```python
from build123d import *

# Parameters (mm, degrees)
F0_R = 2.5
F2_R = 1.5
F5_R = 1.5
F8_R = 1


with BuildPart() as f3:
    # F0 (on Top) → F3 section 0
    with BuildSketch(Plane.XY):
        Circle(F0_R)
    # F2 (on offset) → F3 section 1
    with BuildSketch(Plane.XY.offset(8)):
        Circle(F2_R)
    loft()

    # F7: sweep along a path in F6
    with BuildLine(Plane.XZ) as f7_path:
        ThreePointArc((3.5, 10.7476860285), (1.5570925767, 9.9429074233), (0.7523139715, 8))
    # F5 (on offset) → F7 (sweep)
    with BuildSketch(Plane.YZ.offset(3.5)):
        with Locations((0, 11.5)):
            Circle(F5_R)
    sweep(path=f7_path.line)

    # F8
    f8_edges = [f3.edges().sort_by_distance(p)[0] for p in [
        (-1.06066, -1.06066, 8),
    ]]
    fillet(f8_edges, radius=F8_R)


solid = f3.part
```
Work out the finished part from the listing and answer in its coordinate system (mm). Give positions to 0.01 mm unless a question says otherwise; leave off trailing zeros. Order: outer loops, then holes, each group sorted by start corner. A loop starts at its lowest first (then second) coordinate and runs counter-clockwise, first axis right, second up. Notation, with made-up numbers: M 9,-9 L 41,-9 A26 ccw 41,21 Z; hole C 28,20.5 d5. An arc over 180 degrees is marked long. Return JSON: item names as keys, results as strings.
1) For a pull along Z with two mould halves and no side action, classify faces 1 (the flat face through (3.5, 0, 11)), 2 (the flat face through (0, 0, 0)), 3 (the conical face through (0, -2, 4)) as +Z half, -Z half, draft (parallel to the pull), parting line (faces both ways), or undercut.
Resolved:
{"face 1": "draft", "face 2": "-Z half", "face 3": "undercut"}
2) Section A-A, the plane z = 6.5 is taken. Write down the section's boundary in (x, y) (1 decimal), plus the area to 3 significant figures.
Resolved:
{"outline": "C 0,0 d3.4", "area": "8.95 mm^2"}
3) Each of these flat-tipped pins is pushed along its axis until it touches: pin 1 (2 mm diameter, centred on x = 0, z = 10, fed in from +Y); pin 2 (1 mm diameter, centred on y = 0, z = 7, fed in from -X); pin 3 (1.5 mm diameter, centred on x = 0.5, z = 4, fed in from -Y). Where does it stop, or does it pass through?
Resolved:
{"pin 1": "y = 1.5", "pin 2": "x = -1.69", "pin 3": "y = -2.08"}
4) Section B-B, the plane z = 1 is taken. Write down the section's boundary in (x, y) (3 decimals), plus the area to 3 significant figures.
Resolved:
{"outline": "C 0,0 d4.75", "area": "17.7 mm^2"}
5) Straight lines are drawn through the part: line 1 along Y through (x, z) = (0.5, 10); line 2 along Y through (x, z) = (-1.25, 1.75); line 3 along X through (y, z) = (0.8, 8.25). For each, find the intervals that lie inside material, in ascending order. Write a range as [from, to].
Resolved:
{"line 1": "[-1.5, 1.5]", "line 2": "[-1.91, 1.91]", "line 3": "[-1.26, 1.28]"}
